Verification items for the finished model (mm, model axes). A direction names the side the tool comes from. Give positions to 0.01 mm unless a question says otherwise; leave off trailing zeros. Write each loop counter-clockwise with the first axis right and the second up, starting at its lowest first coordinate (ties: lowest second). Pieces come first, ordered by that corner, then holes. Notation, with made-up numbers: M 18.25,21 L 31.25,21 A12 ccw 31.25,30 Z; hole C 77,13 d2. An arc over 180 degrees is marked long. Write item = value, one per line.
from build123d import *

# Parameters (mm, degrees)
PAD_DEPTH       = 22
POCKET_DEPTH    = 4
POCKET001_DEPTH = 19


with BuildPart() as part:
    # Sketch009 → Pad (new body)
    with BuildSketch(Plane.XY):
        with BuildLine():
            Line((-32.90217, 117.6749), (49.38771, 117.6749))
            ThreePointArc((106.745131, 114.51814), (78.109822, 116.885113), (49.38771, 117.6749))
            ThreePointArc((126.84683, 92.07491), (121.086688, 107.139578), (106.745131, 114.51814))
            Line((126.84683, 16.22193), (126.84683, 92.07491))
            ThreePointArc((106.09683, -4.52807), (120.769296, 1.549464), (126.84683, 16.22193))
            Line((78.817048, -4.52807), (106.09683, -4.52807))
            ThreePointArc((58.97856, -19.25), (71.330694, -15.167467), (78.817048, -4.52807))
            Line((5.169501, -19.25), (58.97856, -19.25))
            Line((-3.90385, -24.50197), (5.169501, -19.25))
            ThreePointArc((-31.01326, -17.365921), (-18.929599, -26.522348), (-3.90385, -24.50197))
            Line((-44.46621, 5.526299), (-31.01326, -17.365921))
            ThreePointArc((-55.481775, 44.57846), (-52.490743, 24.342472), (-44.46621, 5.526299))
            Line((-55.481775, 95.095295), (-55.481775, 44.57846))
            ThreePointArc((-32.90217, 117.6749), (-48.868362, 111.061487), (-55.481775, 95.095295))
        make_face()
    extrude(amount=-PAD_DEPTH)

    # Sketch010 → Pocket (cut)
    with BuildSketch(Plane.XY):
        with BuildLine():
            Line((49.38771, 106.4249), (-32.899678, 106.4249))
            ThreePointArc((-32.899678, 106.4249), (-40.910919, 103.106535), (-44.229283, 95.095295))
            Line((-44.229283, 95.095295), (-44.229283, 44.57846))
            ThreePointArc((-44.229283, 44.57846), (-41.906554, 27.194286), (-35.101321, 11.029714))
            Line((-21.648371, -11.862506), (-35.101321, 11.029714))
            ThreePointArc((-21.648371, -11.862506), (-16.164503, -16.017921), (-9.345444, -15.101023))
            Line((2.252489, -8.387738), (-9.345444, -15.101023))
            Line((58.97856, -8.387738), (2.252489, -8.387738))
            ThreePointArc((58.97856, -8.387738), (65.954415, -5.498245), (68.843908, 1.47761))
            Line((68.843908, 6.72193), (68.843908, 1.47761))
            Line((106.09683, 6.72193), (68.843908, 6.72193))
            ThreePointArc((106.09683, 6.72193), (112.814344, 9.504416), (115.59683, 16.22193))
            Line((115.59683, 92.07491), (115.59683, 16.22193))
            ThreePointArc((115.59683, 92.07491), (112.706605, 99.633799), (105.510546, 103.336087))
            ThreePointArc((105.510546, 103.336087), (77.491595, 105.652113), (49.38771, 106.4249))
        make_face()
    extrude(amount=-POCKET_DEPTH, mode=Mode.SUBTRACT)

    # Sketch011 → Pocket001 (cut)
    with BuildSketch(Plane.XY):
        with BuildLine():
            Line((-37.227702, 99.4249), (49.38771, 99.4249))
            ThreePointArc((104.74236, 96.378365), (77.106921, 98.66269), (49.38771, 99.4249))
            ThreePointArc((108.59683, 92.07491), (107.492332, 94.963537), (104.74236, 96.378365))
            Line((108.59683, 16.22193), (108.59683, 92.07491))
            ThreePointArc((106.09683, 13.72193), (107.864597, 14.454163), (108.59683, 16.22193))
            Line((61.45617, 13.72193), (106.09683, 13.72193))
            Line((61.45617, 1.47761), (61.45617, 13.72193))
            ThreePointArc((58.97856, -1), (60.730495, -0.274325), (61.45617, 1.47761))
            Line((0.268545, -1), (58.97856, -1))
            Line((-13.046428, -8.707168), (0.268545, -1))
            ThreePointArc((-15.279039, -8.119475), (-14.283882, -8.873557), (-13.046428, -8.707168))
            Line((-28.731989, 14.772745), (-15.279039, -8.119475))
            ThreePointArc((-37.227702, 44.57846), (-34.879927, 29.13401), (-28.731989, 14.772745))
            Line((-37.227702, 99.4249), (-37.227702, 44.57846))
        make_face()
    extrude(amount=-POCKET001_DEPTH, mode=Mode.SUBTRACT)


solid = part.part
1) Cross-section at B-B on y = 85.5. Record the boundary of the cut face in (x, z).
From the geometry:
outline = M -55.48,-22 L 126.85,-22 L 126.85,0 L 115.6,0 L 115.6,-4 L 108.6,-4 L 108.6,-19 L -37.23,-19 L -37.23,-4 L -44.23,-4 L -44.23,0 L -55.48,0 Z
2) Material ranges on probe 1 along Y at (x, z) = (51.5, -6.75); probe 2 along X at (y, z) = (48.5, -14.5); probe 3 along Z at (x, y) = (-12.5, 22.5), recorded low to high. Write a range as from..to.
From the geometry:
probe_1 = -19.25..-1, 99.42..117.67
probe_2 = -55.48..-37.23, 108.6..126.85
probe_3 = -22..-19
3) Draft check along Y on faces 3 (the flat face through (36, 115, 0)), 4 (the cylindrical face through (112.74, 9.43, -1.97)), 5 (the cylindrical face through (78.512, 116.863, -10.846)). Enter one of: +Y half, -Y half, draft (parallel to the pull), parting line (faces both ways), or undercut.
From the geometry:
face_3 = draft
face_4 = undercut
face_5 = +Y half
4) Cross-section at C-C on x = 15.5. Record the boundary of the cut face in (y, z).
From the geometry:
outline = M -19.25,-22 L 117.67,-22 L 117.67,0 L 106.42,0 L 106.42,-4 L 99.42,-4 L 99.42,-19 L -1,-19 L -1,-4 L -8.39,-4 L -8.39,0 L -19.25,0 Z
5) Tool access check on faces 1 (the cylindrical face through (77.88, 105.63, -1.97)), 2 (the cylindrical face through (121.24, 106.967, -10.846)). Record the directions out of +Z, -Z, +X, -X, +Y, -Y that give a thin tool (end or side, any length) a straight path to the whole face; none if there is none.
From the geometry:
face_1 = +Z
face_2 = +Z, -Z, +X, +Y
6) Cross-section at D-D on x = -41. Record the boundary of the cut face in (y, z), plus the area to 3 significant figures.
From the geometry:
outline = M -0.37,-22 L 116.17,-22 L 116.17,0 L 103.02,0 L 103.02,-4 L 24.15,-4 L 24.15,0 L -0.37,0 Z
area = 2,250 mm^2
7) Cross-section at A-A on z = -7.25. Record the boundary of the cut face in (x, y).
From the geometry:
outline = M -55.48,44.58 A80.01 ccw -44.47,5.53 L -31.01,-17.37 A19.89 ccw -3.9,-24.5 L 5.17,-19.25 L 58.98,-19.25 A20.73 ccw 78.82,-4.53 L 106.1,-4.53 A20.75 ccw 126.85,16.22 L 126.85,92.07 A22.58 ccw 106.75,114.52 A522.66 ccw 49.39,117.67 L -32.9,117.67 A22.58 ccw -55.48,95.1 Z; hole M -37.23,44.58 A61.76 ccw -28.73,14.77 L -15.28,-8.12 A1.64 ccw -13.05,-8.71 L 0.27,-1 L 58.98,-1 A2.48 ccw 61.46,1.48 L 61.46,13.72 L 106.1,13.72 A2.5 ccw 108.6,16.22 L 108.6,92.07 A4.33 ccw 104.74,96.38 A504.41 ccw 49.39,99.42 L -37.23,99.42 Z
8) Depth check by flat-ended pin: P1, Ø6.5, axis at x = 91, z = -14, coming from the -Y side; P2, Ø1, axis at y = 103, z = -7.5, coming from the -X side; P3, Ø4.5, axis at x = -10, z = -3, coming from the -Y side. Enter the tip coordinate at first touch or a pass-through.
From the geometry:
P1 = -4.53
P2 = -54.23
P3 = -27.11
